Autodesk Inventor part; units mm, degrees
ref_plane "YZ Plane" through (0, 0, 0) normal (1, 0, 0) x (0, 1, 0)
ref_plane "XZ Plane" through (0, 0, 0) normal (0, 1, 0) x (-1, 0, 0)
ref_plane "XY Plane" through (0, 0, 0) normal (0, 0, 1) x (1, 0, 0)
sketch "Sketch1" plane through (0, 0, 0) normal (0, 0, 1) x (1, 0, 0)
  circle A0 centre (0, 0) radius 2.5
  dimension "d0" = 5
extrude "Extrusion1" add sketch "Sketch1" along normal blind 10
sketch "Sketch2" plane through (0, 0, 10) normal (0, 0, 1) x (1, 0, 0)
  line L0 (-1.45, 1.45) -> (1.45, 1.45)
  line L1 (1.45, 1.45) -> (1.45, -1.45)
  line L2 (1.45, -1.45) -> (-1.45, -1.45)
  line L3 (-1.45, -1.45) -> (-1.45, 1.45)
  line L4 (-1.45, 1.45) -> (1.45, -1.45) construction
  line L5 (1.45, 1.45) -> (-1.45, -1.45) construction
  point P0 (0, 0)
  dimension "d3" = 2.9
extrude "Extrusion2" add sketch "Sketch2" along normal blind 10
properties part number "MINI Stepper Shaft ( Pinion )"
CAD build for the part. Positions are in the model's coordinates, mm. A direction names the side the tool comes from. Round coordinates to 2 decimals unless told otherwise and drop trailing zeros. Loops run counter-clockwise (first coordinate to the right, second up) from the corner with the lowest first, then second, coordinate; pieces in that order, holes last. Notation, with made-up numbers: M -13.5,36 L 43.5,36 A24 cw 43.5,65 Z; hole C 44,71 d1. An arc over 180 degrees is marked long. Use a Markdown table: item, result. Add a question column.
(1) Pull direction Y, two halves, no side cores. Call faces 4 (the face through (0, 1.45, 15)), 5 (the face through (1.45, 0, 15)), 6 (the face through (-0.54, 2.44, 4.93)): +Y half, -Y half, draft (parallel to the pull), parting line (faces both ways), or undercut.
(2) Cut at B-B (y = 0.4). Give the cut face in (x, z), and give its area (3 significant figures).
(3) Cut at A-A (x = 0). Give the cut face in (y, z), and give its area (3 significant figures).
(4) Cut at D-D (z = 17.25). Give the cut face in (x, y), and give its area (3 significant figures).
(5) Flat gauge pins, fed straight in: pin 1 (1.5 mm diameter, centred on y = 0, z = 14.5, fed in from -X); pin 2 (3 mm diameter, centred on x = 0.5, z = 15, fed in from -Y); pin 3 (3 mm diameter, centred on y = 0, z = 13.5, fed in from +X). Where does each tip first touch, or does it go through?
(6) Cut at C-C (z = 6.5). Give the cut face in (x, y).
(7) Drill centre lines: line 1 (Y direction, x = 0.75, z = 10.5); line 2 (Z direction, x = 0.05, y = -1.65). Where is each one in solid material? Low to high.
(8) Which spindle directions (+Z, -Z, +X, -X, +Y, -Y) get a long thin tool onto all of the face, cutting with end or side? Do faces 1 (the face through (-1.45, 0, 15)), 2 (the face through (0, -1.45, 15)), 3 (the face through (0, 0, 20)). Say none if no direction does.
Geometry says:
| question | item | result |
|---|---|---|
| 1 | face 4 | +Y half |
| 1 | face 5 | draft |
| 1 | face 6 | parting line |
| 2 | outline | M -2.47,0 L 2.47,0 L 2.47,10 L 1.45,10 L 1.45,20 L -1.45,20 L -1.45,10 L -2.47,10 Z |
| 2 | area | 78.4 mm² |
| 3 | outline | M -2.5,0 L 2.5,0 L 2.5,10 L 1.45,10 L 1.45,20 L -1.45,20 L -1.45,10 L -2.5,10 Z |
| 3 | area | 79.0 mm² |
| 4 | outline | M -1.45,-1.45 L 1.45,-1.45 L 1.45,1.45 L -1.45,1.45 Z |
| 4 | area | 8.41 mm² |
| 5 | pin 1 | stops at x = -1.45 |
| 5 | pin 2 | stops at y = -1.45 |
| 5 | pin 3 | stops at x = 1.45 |
| 6 | outline | C 0,0 d5 |
| 7 | line 1 | y = -1.45 to 1.45 |
| 7 | line 2 | z = 0 to 10 |
| 8 | face 1 | +Z, -X, +Y, -Y |
| 8 | face 2 | +Z, +X, -X, -Y |
| 8 | face 3 | +Z, +X, -X, +Y, -Y |
